from build123d import *

# Parameters (mm, degrees)
F0_W        = 76.2
F0_H        = 6.35
F1_DEPTH    = 76.2
F2_W        = 25.4
F2_H        = 25.4
F3_DEPTH    = 25.4
F4_W        = 25.4
F4_H        = 3.5260361671
F5_DEPTH    = 5.08
F8_T1_DEPTH = 25.4


# Not quite as in the source:
# - a fillet or chamfer that OpenCascade refuses, or shapes differently, is made with other operations: its cross-section is extruded or revolved along the edge and cut away or added
# - the program builds the solid bodies; features that only make, move or delete a surface that nothing else refers to are left out


with BuildPart() as f1:
    # F0 (on Top) → F1 (new body)
    with BuildSketch(Plane.XY):
        Rectangle(F0_W, F0_H)
    extrude(amount=F1_DEPTH)

    # F2 (on face) → F3 (cut)
    with BuildSketch(Plane.XZ.offset(3.175)):
        with Locations((0, 38.1)):
            Rectangle(F2_W, F2_H)
    extrude(amount=-F3_DEPTH, mode=Mode.SUBTRACT)

    # F4 (on face) → F5 (cut)
    with BuildSketch(Plane.XZ.offset(3.175)):
        with Locations((25.4, 39.8630180836)):
            Rectangle(F4_W, F4_H)
    extrude(amount=-F5_DEPTH, mode=Mode.SUBTRACT)

    # F8: fillet of radius 1.778 on 2 edges, made by hand

    # F8_s2 → F8_t1 (join)
    with BuildSketch(Plane.YZ.offset(12.7)):
        with BuildLine():
            ThreePointArc((0.127, 41.6260361671), (1.3842358569, 41.1052720241), (1.905, 39.8480361671))
            Line((1.905, 39.8480361671), (1.905, 41.6260361671))
            Line((1.905, 41.6260361671), (0.127, 41.6260361671))
        make_face()
        with BuildLine():
            ThreePointArc((0.127, 38.1), (1.3842358569, 38.6207641431), (1.905, 39.878))
            Line((1.905, 39.878), (1.905, 38.1))
            Line((1.905, 38.1), (0.127, 38.1))
        make_face()
    extrude(amount=F8_T1_DEPTH)


solid = f1.part
Can you work these out from the model? Positions are in its coordinate system, mm. A direction names the side the tool comes from. Round coordinates to 2 decimals unless told otherwise and drop trailing zeros. Order: outer loops, then holes, each group sorted by start corner. A loop starts at its lowest first (then second) coordinate and runs counter-clockwise, first axis right, second up. Notation, with made-up numbers: (-31.75, -31) -> (-13.75, -31) arc R14 cw to (-13.75, -9) -> close; hole circle Ø10 at (-8.5, 55). An arc over 180 degrees is marked (long way). Write each question's results on one line, items separated by ' | '. Start each with the question number.
Item 1: Thinking about a two-plate mould opening in Z: for faces 1 (the flat face through (-1, -3.175, 54)), 2 (the flat face through (25, -2, 38.1)), 3 (the flat face through (-1, 0, 0)), which applies, +Z half, -Z half, draft (parallel to the pull), parting line (faces both ways), or undercut?
Item 2: Which directions (+Z, -Z, +X, -X, +Y, -Y) give clear straight access to the entire face, cutting with the end or side of a thin tool? Please do faces 4 (the flat face through (-12.7, 0, 38)), 5 (the flat face through (-1, 3.175, 54)), 6 (the flat face through (25, -2, 41.626)).
Item 3: If we section it at D-D, the plane y = -0.75: Write out the boundary of the cut face in (x, z).
Item 4: If we section it at A-A, the plane z = 32.5: Write out the boundary of the cut face in (x, y) (3 decimals).
Item 5: If we section it at C-C, the plane x = 32: Write out the boundary of the cut face in (y, z) (3 decimals).
Item 6: If we section it at B-B, the plane x = -3: Write out the boundary of the cut face in (y, z) (3 decimals).
Item 7: Please list where these lines run through material, in increasing order: L1, parallel to Z at x = 20, y = -1; L2, parallel to Z at x = 7.5, y = 0.75; L3, parallel to X at y = -1.75, z = 47.5.
Results:
1) face 1: draft | face 2: undercut | face 3: -Z half
2) face 4: +Y, -Y | face 5: +Z, -Z, +X, -X, +Y | face 6: +X, -Y
3) outline: (-38.1, 0) -> (38.1, 0) -> (38.1, 38.1) -> (12.7, 38.1) -> (12.7, 25.4) -> (-12.7, 25.4) -> (-12.7, 50.8) -> (12.7, 50.8) -> (12.7, 41.63) -> (38.1, 41.63) -> (38.1, 76.2) -> (-38.1, 76.2) -> close
4) outline: (-38.1, -3.175) -> (-12.7, -3.175) -> (-12.7, 3.175) -> (-38.1, 3.175) -> close; (12.7, -3.175) -> (38.1, -3.175) -> (38.1, 3.175) -> (12.7, 3.175) -> close
5) outline: (-3.175, 0) -> (3.175, 0) -> (3.175, 76.2) -> (-3.175, 76.2) -> (-3.175, 41.626) -> (0.127, 41.626) arc R1.778 cw to (1.905, 39.863) arc R1.778 cw to (0.127, 38.1) -> (-3.175, 38.1) -> close
6) outline: (-3.175, 0) -> (3.175, 0) -> (3.175, 25.4) -> (-3.175, 25.4) -> close; (-3.175, 50.8) -> (3.175, 50.8) -> (3.175, 76.2) -> (-3.175, 76.2) -> close
7) L1: z = 0 to 38.1, 41.63 to 76.2 | L2: z = 0 to 25.4, 50.8 to 76.2 | L3: x = -38.1 to -12.7, 12.7 to 38.1
